from build123d import *

# Parameters (mm, degrees)
F1_DEPTH = 38.1
F2_R     = 5.08
F7_DEPTH = 12.7
F8_DEPTH = 12.7


# Not quite as in the source:
# - a pattern or mirror of a feature is missing from the dataset's text; its kind, count and spacing are read off the source's solid


with BuildPart() as f1:
    # F0 (on Front) → F1 (new body)
    with BuildSketch(Plane.XZ):
        with BuildLine():
            Line((-9.3345, 82.804), (-9.3345, 101.1702876825))
            ThreePointArc((-9.3345, 101.1702876825), (-22.880190841, 98.9901857109), (-36.0086465439, 95.0049334197))
            Line((-36.0086465439, 95.0049334197), (-33.7581061349, 89.067125081))
            ThreePointArc((-33.7581061349, 89.067125081), (-24.8415554365, 91.9535731959), (-15.6845, 93.9497682794))
            Line((-15.6845, 93.9497682794), (-15.6845, 76.454))
            Line((-15.6845, 76.454), (15.6845, 76.454))
            Line((15.6845, 76.454), (15.6845, 93.9497682794))
            ThreePointArc((15.6845, 93.9497682794), (24.8415554365, 91.9535731959), (33.7581061349, 89.067125081))
            Line((33.7581061349, 89.067125081), (36.0086465439, 95.0049334197))
            ThreePointArc((36.0086465439, 95.0049334197), (22.880190841, 98.9901857109), (9.3345, 101.1702876825))
            Line((9.3345, 101.1702876825), (9.3345, 82.804))
            Line((9.3345, 82.804), (-9.3345, 82.804))
        make_face()
    extrude(amount=F1_DEPTH)

    # F2
    f2_edges = [f1.edges().sort_by_distance(p)[0] for p in [
        (-9.3345, -19.05, 101.170288),
        (9.3345, -19.05, 101.170288),
        (15.6845, -19.05, 93.949768),
        (-15.6845, -19.05, 93.949768),
        (15.6845, -19.05, 76.454),
        (-15.6845, -19.05, 76.454),
    ]]
    fillet(f2_edges, radius=F2_R)

    # F4 (on face) → F7 (cut, symmetric)
    with BuildSketch(Plane(origin=(-25.5909022193, 0, 97.7327744919), x_dir=(0.9673862364, 0, 0.2533058814), z_dir=(0.2533058814, 0, -0.9673862364))):
        with BuildLine():
            Line((-1.8789606614, 5.461), (-1.8789606614, 9.779))
            ThreePointArc((-1.8789606614, 9.779), (-4.0379606614, 7.62), (-1.8789606614, 5.461))
        make_face()
    extrude(amount=F7_DEPTH, both=True, mode=Mode.SUBTRACT)

    # F4 (on face) → F8 (cut, symmetric)
    with BuildSketch(Plane(origin=(-25.5909022193, 0, 97.7327744919), x_dir=(0.9673862364, 0, 0.2533058814), z_dir=(0.2533058814, 0, -0.9673862364))):
        with BuildLine():
            ThreePointArc((-1.8789606614, 32.639), (-4.0379606614, 30.48), (-1.8789606614, 28.321))
            Line((-1.8789606614, 28.321), (-1.8789606614, 30.48))
            Line((-1.8789606614, 30.48), (-1.8789606614, 32.639))
        make_face()
        with BuildLine():
            Line((-1.8789606614, 30.48), (-1.8789606614, 28.321))
            ThreePointArc((-1.8789606614, 28.321), (-0.3523171208, 28.9533564594), (0.2800393386, 30.48))
            ThreePointArc((0.2800393386, 30.48), (-0.3523171208, 32.0066435406), (-1.8789606614, 32.639))
            Line((-1.8789606614, 32.639), (-1.8789606614, 30.48))
        make_face()
        with BuildLine():
            ThreePointArc((-1.8789606614, 5.461), (-0.3523171208, 6.0933564594), (0.2800393386, 7.62))
            ThreePointArc((0.2800393386, 7.62), (-0.3523171208, 9.1466435406), (-1.8789606614, 9.779))
            Line((-1.8789606614, 9.779), (-1.8789606614, 5.461))
        make_face()
        with BuildLine():
            Line((-1.8789606614, 5.461), (-1.8789606614, 9.779))
            ThreePointArc((-1.8789606614, 9.779), (-4.0379606614, 7.62), (-1.8789606614, 5.461))
        make_face()
    f8 = extrude(amount=F8_DEPTH, both=True, mode=Mode.SUBTRACT)

    # F8_copies: F8 across plane
    add(f8.mirror(Plane(origin=(6e-06, 0, 0), x_dir=(0, 0, 1), z_dir=(1, 0, 0))), mode=Mode.SUBTRACT)


solid = f1.part
Verification items for the finished model (mm, model axes). A direction names the side the tool comes from. Round coordinates to 2 decimals unless told otherwise and drop trailing zeros. Write each loop counter-clockwise with the first axis right and the second up, starting at its lowest first coordinate (ties: lowest second). Pieces come first, ordered by that corner, then holes.
(1) Section check B-B (y = -35). Enter the section's corners in (x, z).
Returned:
outline: (-36.01, 95) - (-33.76, 89.07) arc R95.25 cw to (-21.93, 92.69) arc R5.08 cw to (-15.68, 87.75) - (-15.68, 81.53) arc R5.08 ccw to (-10.6, 76.45) - (10.6, 76.45) arc R5.08 ccw to (15.68, 81.53) - (15.68, 87.75) arc R5.08 cw to (21.93, 92.69) arc R95.25 cw to (33.76, 89.07) - (36.01, 95) arc R101.6 ccw to (15.17, 100.46) arc R5.08 ccw to (9.33, 95.44) - (9.33, 82.8) - (-9.33, 82.8) - (-9.33, 95.44) arc R5.08 ccw to (-15.17, 100.46) arc R101.6 ccw to start
(2) Access from +Z, -Z, +X, -X, +Y, -Y to the whole of each face (thin tool, end or side, straight path). Record for faces 1 (the cylindrical face through (25.88, -18.78, 98.25)), 2 (the cylindrical face through (-27.988, -18.783, 91.045)), 3 (the flat face through (9.334, -19, 89)), 4 (the flat face through (-15.684, -19, 85)), 5 (the cylindrical face through (-25.59, -18.783, 98.325)).
Returned:
face 1: +Z, +X, +Y, -Y
face 2: -Z, +Y, -Y
face 3: +Z, +Y, -Y
face 4: -Z, -X, +Y, -Y
face 5: +Z, -X, +Y, -Y
(3) Section check A-A (z = 85.5). Enter the section's corners in (x, y).
Returned:
outline: (-15.68, -38.1) - (-9.33, -38.1) - (-9.33, 0) - (-15.68, 0) - close; (9.33, -38.1) - (15.68, -38.1) - (15.68, 0) - (9.33, 0) - close
(4) Material ranges on line 1 (X direction, y = -32.5, z = 84); line 2 (X direction, y = -30, z = 93); line 3 (X direction, y = -31.5, z = 97.5), recorded low to high.
Returned:
line 1: x = -15.68 to -9.33, 9.33 to 15.68
line 2: x = -35.25 to -28.47, -24.12 to -9.33, 9.33 to 24.12, 28.47 to 35.25
line 3: x = -25.51 to -9.77, 9.77 to 25.51
(5) Section check D-D (z = 90.25). Enter the section's corners in (x, y), plus the area to 3 significant figures.
Returned:
outline: (-34.21, -38.1) - (-30.45, -38.1) - (-30.45, 0) - (-34.21, 0) - close; (-16.34, -38.1) - (-9.33, -38.1) - (-9.33, 0) - (-16.34, 0) - close; (9.33, -38.1) - (16.34, -38.1) - (16.34, 0) - (9.33, 0) - close; (30.45, -38.1) - (34.21, -38.1) - (34.21, 0) - (30.45, 0) - close
area: 820 mm2
(6) Mould release check, pull along X, two halves, no side actions. Record for faces 6 (the cylindrical face through (-17.7, -19.3, 91.8)), 7 (the flat face through (-3, -38.1, 82)), 8 (the flat face through (-34.9, -18.78, 92.08)), 9 (the flat face through (15.684, -19, 85)): pulls with the +X half, pulls with the -X half, needs draft (parallel to the pull), parting line crosses it, or undercut.
Returned:
face 6: undercut
face 7: needs draft
face 8: pulls with the -X half
face 9: pulls with the +X half
(7) Section check C-C (y = -8.5). Enter the section's corners in (x, z).
Returned:
outline: (-36.01, 95) - (-33.76, 89.07) arc R95.25 cw to (-27.83, 91.09) - (-29.44, 97.24) arc R101.6 ccw to start; (-25.65, 98.31) - (-24.04, 92.17) arc R95.25 cw to (-21.93, 92.69) arc R5.08 cw to (-15.68, 87.75) - (-15.68, 81.53) arc R5.08 ccw to (-10.6, 76.45) - (10.6, 76.45) arc R5.08 ccw to (15.68, 81.53) - (15.68, 87.75) arc R5.08 cw to (21.93, 92.69) arc R95.25 cw to (24.04, 92.17) - (25.65, 98.31) arc R101.6 ccw to (15.17, 100.46) arc R5.08 ccw to (9.33, 95.44) - (9.33, 82.8) - (-9.33, 82.8) - (-9.33, 95.44) arc R5.08 ccw to (-15.17, 100.46) arc R101.6 ccw to start; (27.83, 91.09) arc R95.25 cw to (33.76, 89.07) - (36.01, 95) arc R101.6 ccw to (29.44, 97.24) - close
(8) Depth check by flat-ended pin: pin 1 Ø2 at (x, y) = (17.5, -23.5) entering from +Z; pin 2 Ø4 at (y, z) = (-10, 84) entering from +X; pin 3 Ø8 at (x, z) = (11.5, 85) entering from +Y; pin 4 Ø8 at (x, y) = (-24.5, -31) entering from -Z. Enter the tip coordinate at first touch or a pass-through.
Returned:
pin 1: stops at z = 100.25
pin 2: stops at x = 15.68
pin 3: stops at y = 0
pin 4: stops at z = 90.89
